For this review, take the finished solid that the model builds, in its own axes (mm). A direction names the side the tool comes from. Give positions to 0.01 mm unless a question says otherwise; leave off trailing zeros. Order: outer loops, then holes, each group sorted by start corner. A loop starts at its lowest first (then second) coordinate and runs counter-clockwise, first axis right, second up. Notation, with made-up numbers: (-40, 4.5) -> (12, 4.5) arc R19 cw to (12, 38.5) -> close; hole circle Ø9 at (-22, -15). An arc over 180 degrees is marked (long way). Return JSON: item names as keys, results as strings. Group by question number.
1) For faces 5 (the face through (-32.438, -38.024, 98.514)), 6 (the face through (-4.445, -102, -27)), 7 (the face through (-1.29, -133.26, 101.69)), list the 3-axis set-ups (+Z, -Z, +X, -X, +Y, -Y) from which the entire face can be reached by the end or side of a thin tool; tool diameter is ignored.
2) Add section A-A (x = 82.55). Give the boundary of the cut face in (y, z) (3 decimals), then the cut area to 3 significant figures.
3) The part is to be moulded in two halves that separate along X. For faces 1 (the face through (32, -35, 92.075)), 2 (the face through (-96.45, 55.28, 12.61)), 3 (the face through (-1.29, -133.26, 12.61)), 4 (the face through (101.153, 59.681, 56.617)), say which applies: released by +X, released by -X, zero draft, split by the parting line, or undercut.
4) Add section B-B (y = -101.6). Give the boundary of the cut face in (x, z) (3 decimals).
5) Add section C-C (z = -20). Give the boundary of the cut face in (x, y).
6) To check wall thickness, follow line 1 along Y through (x, z) = (0, 3.5); line 2 along X through (y, z) = (25, 5) (3 decimals); line 3 along Y through (x, z) = (82.55, 86) (3 decimals). State the ranges of each line that lie inside material, in increasing order.
7) Insertion check: P1, Ø5, axis at x = -32.5, y = -8, coming from the +Z side (3 decimals); P2, Ø2, axis at x = -4, y = -95, coming from the -Z side; P3, Ø1.6, axis at x = 4.5, z = 106.5, coming from the +Y side. Each pin has a flat end and moves straight along its axis. Give the tip position at first contact, or say it passes through.
from build123d import *

# Parameters (mm, degrees)
SKETCH1_W           = 158.75
SKETCH1_H           = 50.8
SKETCH1_R           = 1.5875
BOSS_EXTRUDE1_DEPTH = 6.35
BOSS_EXTRUDE2_DEPTH = 101.6
CHAMFER1_SIZE       = 12.7
SKETCH3_R           = 3.175
CUT_EXTRUDE3_DEPTH  = 31.75
CUT_EXTRUDE4_DEPTH  = 3.175
SKETCH5_R           = 3.175
CUT_EXTRUDE5_DEPTH  = 12.7
SKETCH6_R           = 6.35
BOSS_EXTRUDE3_DEPTH = 29.845
BOSS_EXTRUDE4_DEPTH = 6.35
SKETCH8_R           = 6.35
BOSS_EXTRUDE5_DEPTH = 12.7


with BuildPart() as part:
    # Sketch1 → Boss-Extrude1 (new body)
    with BuildSketch(Plane.XY):
        with Locations((0, 25.4)):
            Rectangle(SKETCH1_W, SKETCH1_H)
        with Locations((53.975, 38.1)):
            Circle(SKETCH1_R, mode=Mode.SUBTRACT)
        with Locations(Location((53.975, 12.7, 0), (0, 0, 180))):
            Circle(SKETCH1_R, mode=Mode.SUBTRACT)
        with Locations((-53.975, 12.7)):
            Circle(SKETCH1_R, mode=Mode.SUBTRACT)
        with Locations(Location((-53.975, 38.1, 0), (0, 0, 180))):
            Circle(SKETCH1_R, mode=Mode.SUBTRACT)
        with Locations((0, 25.4)):
            Circle(SKETCH1_R, mode=Mode.SUBTRACT)
    extrude(amount=BOSS_EXTRUDE1_DEPTH)

    # Sketch2 → Boss-Extrude2 (add)
    with BuildSketch(Plane.XY.offset(6.35)):
        with BuildLine():
            Line((-92.075, -139.7), (92.075, -139.7))
            ThreePointArc((92.075, -139.7), (101.055256121, -135.980256121), (104.775, -127))
            Line((104.775, -127), (104.775, 50.8))
            ThreePointArc((104.775, 50.8), (101.055256121, 59.780256121), (92.075, 63.5))
            Line((92.075, 63.5), (-92.075, 63.5))
            ThreePointArc((-92.075, 63.5), (-101.055256121, 59.780256121), (-104.775, 50.8))
            Line((-104.775, 50.8), (-104.775, -127))
            ThreePointArc((-104.775, -127), (-101.055256121, -135.980256121), (-92.075, -139.7))
        make_face()
    extrude(amount=BOSS_EXTRUDE2_DEPTH)

    # Chamfer1
    chamfer1_edges = [part.edges().sort_by_distance(p)[0] for p in [
        (-101.055256121, -135.980256121, 6.35),
        (0, -139.7, 6.35),
        (101.055256121, -135.980256121, 6.35),
        (104.775, -38.1, 6.35),
        (101.055256121, 59.780256121, 6.35),
        (0, 63.5, 6.35),
        (-101.055256121, 59.780256121, 6.35),
        (-104.775, -38.1, 6.35),
        (-101.055256121, -135.980256121, 107.95),
        (0, -139.7, 107.95),
        (101.055256121, -135.980256121, 107.95),
        (104.775, -38.1, 107.95),
        (101.055256121, 59.780256121, 107.95),
        (0, 63.5, 107.95),
        (-101.055256121, 59.780256121, 107.95),
        (-104.775, -38.1, 107.95),
    ]]
    chamfer(chamfer1_edges, length=CHAMFER1_SIZE - 0.0001)  # a hair under: the kernel refuses the full size

    # Sketch3 → Cut-Extrude3 (cut)
    with BuildSketch(Plane.XY.offset(107.95)):
        with Locations((-82.55, -6.35)):
            Circle(SKETCH3_R)
        with Locations(Location((-82.55, -69.85, 0), (0, 0, 180))):
            Circle(SKETCH3_R)
        with Locations((82.55, -69.85)):
            Circle(SKETCH3_R)
        with Locations(Location((82.55, -6.35, 0), (0, 0, 180))):
            Circle(SKETCH3_R)
    extrude(amount=-CUT_EXTRUDE3_DEPTH, mode=Mode.SUBTRACT)

    # Sketch4 → Cut-Extrude4 (cut)
    with BuildSketch(Plane.XY.offset(107.95)):
        with BuildLine():
            Line((50.8, 12.7), (-50.8, 12.7))
            ThreePointArc((-50.8, 12.7), (-55.869513916, 10.173941508), (-56.905677068, 4.605520838))
            Line((-56.905677068, 4.605520838), (-44.205677068, -39.844479162))
            ThreePointArc((-44.205677068, -39.844479162), (-41.923941508, -43.169513916), (-38.1, -44.45))
            Line((-38.1, -44.45), (38.1, -44.45))
            ThreePointArc((38.1, -44.45), (41.923941508, -43.169513916), (44.205677068, -39.844479162))
            Line((44.205677068, -39.844479162), (56.905677068, 4.605520838))
            ThreePointArc((56.905677068, 4.605520838), (55.869513916, 10.173941508), (50.8, 12.7))
        make_face()
    extrude(amount=-CUT_EXTRUDE4_DEPTH, mode=Mode.SUBTRACT)

    # Sketch5 → Cut-Extrude5 (cut)
    with BuildSketch(Plane.XY.offset(104.775)):
        with Locations((-31.75, 3.175)):
            Circle(SKETCH5_R)
        with Locations((-31.75, -9.525)):
            Circle(SKETCH5_R)
        with Locations((-31.75, -22.225)):
            Circle(SKETCH5_R)
        with Locations((-31.75, -34.925)):
            Circle(SKETCH5_R)
        with Locations(Location((31.75, -34.925, 0), (0, 0, 180))):
            Circle(SKETCH5_R)
        with Locations(Location((31.75, -22.225, 0), (0, 0, 180))):
            Circle(SKETCH5_R)
        with Locations(Location((31.75, -9.525, 0), (0, 0, 180))):
            Circle(SKETCH5_R)
        with Locations(Location((31.75, 3.175, 0), (0, 0, 180))):
            Circle(SKETCH5_R)
    extrude(amount=-CUT_EXTRUDE5_DEPTH, mode=Mode.SUBTRACT)

    # Sketch6 → Boss-Extrude3 (add)
    with BuildSketch(Plane(origin=(0, 0, 6.35), x_dir=(-1, 0, 0), z_dir=(0, 0, -1))):
        with Locations(Location((0, -101.6, 0), (0, 0, 180))):
            Circle(SKETCH6_R)
    extrude(amount=BOSS_EXTRUDE3_DEPTH)

    # Sketch7 → Boss-Extrude4 (add)
    with BuildSketch(Plane(origin=(0, 0, -23.495), x_dir=(-1, 0, 0), z_dir=(0, 0, -1))):
        with BuildLine():
            Line((-4.445, -106.134807052), (4.445, -106.134807052))
            Line((4.445, -106.134807052), (4.445, -97.065192948))
            ThreePointArc((4.445, -97.065192948), (-4.534807052, -97.155), (-4.445, -106.134807052))
        make_face()
    extrude(amount=BOSS_EXTRUDE4_DEPTH)

    # Sketch8 → Boss-Extrude5 (add)
    with BuildSketch(Plane(origin=(0, 0, -29.845), x_dir=(-1, 0, 0), z_dir=(0, 0, -1))):
        with Locations((0, -101.6)):
            Circle(SKETCH8_R)
    extrude(amount=BOSS_EXTRUDE5_DEPTH)


solid = part.part
Evaluation:
{
 "1": {"face 5": "+Z", "face 6": "-X, +Y, -Y", "face 7": "+Z, +X, -X, -Y"},
 "2": {"outline": "(-139.7, 19.05) -> (-127, 6.35) -> (50.8, 6.35) -> (63.5, 19.05) -> (63.5, 95.25) -> (50.8, 107.95) -> (-3.175, 107.95) -> (-3.175, 76.2) -> (-9.525, 76.2) -> (-9.525, 107.95) -> (-66.675, 107.95) -> (-66.675, 76.2) -> (-73.025, 76.2) -> (-73.025, 107.95) -> (-127, 107.95) -> (-139.7, 95.25) -> close", "area": "19,900 mm^2"},
 "3": {"face 1": "undercut", "face 2": "released by -X", "face 3": "zero draft", "face 4": "released by +X"},
 "4": {"outline": "(-104.775, 19.05) -> (-92.075, 6.35) -> (-6.35, 6.35) -> (-6.35, -23.495) -> (-4.445, -23.495) -> (-4.445, -29.845) -> (-6.35, -29.845) -> (-6.35, -42.545) -> (6.35, -42.545) -> (6.35, 6.35) -> (92.075, 6.35) -> (104.775, 19.05) -> (104.775, 95.25) -> (92.075, 107.95) -> (-92.075, 107.95) -> (-104.775, 95.25) -> close"},
 "5": {"outline": "circle Ø12.7 at (0, -101.6)"},
 "6": {"line 1": "-107.95 to -95.25, 0 to 23.81, 26.99 to 50.8", "line 2": "-79.375 to -1.536, 1.536 to 79.375", "line 3": "-139.7 to -73.025, -66.675 to -9.525, -3.175 to 63.5"},
 "7": {"P1": "z = 104.775", "P2": "z = 6.35", "P3": "y = 53.05"}
}
